Model file for the job. Use its own axes, mm. Face numbers are marked on the shaded views. A direction names the side the tool comes from. Round coordinates to 2 decimals unless told otherwise and drop trailing zeros. Loops run counter-clockwise (first coordinate to the right, second up) from the corner with the lowest first, then second, coordinate; pieces in that order, holes last. Notation, with made-up numbers: M 2.25,-11 L 42.25,-11 A25 cw 42.25,12 Z; hole C 10.25,67.5 d9. An arc over 180 degrees is marked long. Answer in a Markdown table with one row per item.
from build123d import *

# Parameters (mm, degrees)
F1_DEPTH = 57
F2_W     = 19
F2_H     = 19
F3_DEPTH = 38
F4_W     = 74
F4_H     = 17.495044
F5_DEPTH = 19
F6_W     = 40
F6_H     = 19
F7_DEPTH = 0.5


with BuildPart() as f1:
    # F0 (on Front) → F1 (new body)
    with BuildSketch(Plane.XZ):
        Polygon((-56, 0), (0, 0), (56, 0), (56, 51), (37, 51), (37, 14.504956), (-37, 14.504956), (-37, 51), (-56, 51), align=None)
    extrude(amount=F1_DEPTH)

    # F2 (on face) → F3 (join)
    with BuildSketch(Plane(origin=(0, 0, 0), x_dir=(-1, 0, 0), z_dir=(0, 1, 0))):
        with Locations((27.5, 24.004956)):
            Rectangle(F2_W, F2_H)
        with Locations((-27.5, 24.004956)):
            Rectangle(F2_W, F2_H)
    extrude(amount=-F3_DEPTH)

    # F4 (on face) → F5 (join)
    with BuildSketch(Plane(origin=(0, 0, 0), x_dir=(-1, 0, 0), z_dir=(0, 1, 0))):
        with Locations((0, 42.252478)):
            Rectangle(F4_W, F4_H)
    extrude(amount=-F5_DEPTH)

    # F6 (on face) → F7 (join, symmetric)
    with BuildSketch(Plane(origin=(0, 0, 0), x_dir=(-1, 0, 0), z_dir=(0, 1, 0))):
        with Locations((-1.049917, 24.004956)):
            Rectangle(F6_W, F6_H)
    extrude(amount=F7_DEPTH, both=True)


solid = f1.part
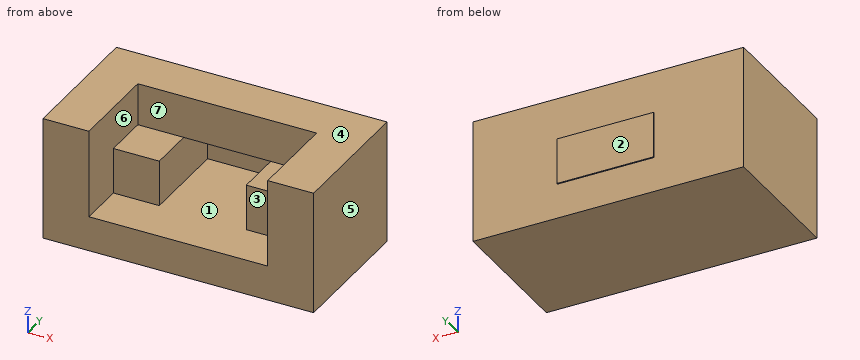
1. Saw through at D-D (y = -15). Write the cut outline in (x, z), and give its area (3 significant figures).
Verdict:
| item | result |
|---|---|
| outline | M -56,0 L 56,0 L 56,51 L -56,51 Z; hole M -18,14.5 L 18,14.5 L 18,33.5 L -18,33.5 Z |
| area | 5,030 mm² |
2. Pin check, flat tips, straight feed: pin 1 (8 mm diameter, centred on x = 14.5, z = 21.5, fed in from -Y); pin 2 (2 mm diameter, centred on x = -16, z = 12.5, fed in from +Y); pin 3 (15 mm diameter, centred on x = -26, y = -28.5, fed in from +Z). Stop position of each tip, or through.
Verdict:
| item | result |
|---|---|
| pin 1 | stops at y = -38 |
| pin 2 | stops at y = 0 |
| pin 3 | stops at z = 33.5 |
3. Mould opens along X. For the marked faces 4, 5, 6 and 7 say: +X half, -X half, draft (parallel to the pull), parting line (faces both ways), or undercut.
Verdict:
| item | result |
|---|---|
| face 4 | draft |
| face 5 | +X half |
| face 6 | undercut |
| face 7 | undercut |
4. Wall check: probe 1 along X at (y, z) = (-53, 31); probe 2 along X at (y, z) = (-31, 19); probe 3 along Z at (x, y) = (10.5, -12.5). Give the ranges that are in metal, low to high.
Verdict:
| item | result |
|---|---|
| probe 1 | x = -56 to -37, 37 to 56 |
| probe 2 | x = -56 to -18, 18 to 56 |
| probe 3 | z = 0 to 14.5, 33.5 to 51 |
5. Tool access for the marked faces 1, 2 and 3: list every direction of +Z, -Z, +X, -X, +Y, -Y with a clear straight run to the whole face (end or side of a thin tool).
Verdict:
| item | result |
|---|---|
| face 1 | -Y |
| face 2 | +Z, -Z, +X, -X, +Y |
| face 3 | +Z, -Y |
6. Saw through at C-C (z = 39). Write the cut outline in (x, y), and give its area (3 significant figures).
Verdict:
| item | result |
|---|---|
| outline | M -56,-57 L -37,-57 L -37,-19 L 37,-19 L 37,-57 L 56,-57 L 56,0 L -56,0 Z |
| area | 3,570 mm² |
7. Saw through at A-A (y = -25.5). Write the cut outline in (x, z).
Verdict:
| item | result |
|---|---|
| outline | M -56,0 L 56,0 L 56,51 L 37,51 L 37,33.5 L 18,33.5 L 18,14.5 L -18,14.5 L -18,33.5 L -37,33.5 L -37,51 L -56,51 Z |
8. Saw through at B-B (x = 4.5). Write the cut outline in (y, z), and give its area (3 significant figures).
Verdict:
| item | result |
|---|---|
| outline | M -57,0 L 0,0 L 0,14.5 L 0.5,14.5 L 0.5,33.5 L 0,33.5 L 0,51 L -19,51 L -19,33.5 L -0.5,33.5 L -0.5,14.5 L -57,14.5 Z |
| area | 1,180 mm² |
